Could you check a few things on this model? Use its own coordinates, in mm. A direction names the side the tool comes from. Give positions to 0.01 mm unless a question says otherwise; leave off trailing zeros. Loops run counter-clockwise (first coordinate to the right, second up) from the corner with the lowest first, then second, coordinate; pieces in that order, holes last. Notation, with made-up numbers: M 48.25,43 L 67.25,43 A21 ccw 67.25,69 Z; hole C 18.25,8 d11. An arc over 180 degrees is marked long. Use a Markdown table: item, result. Add a question column.
1) Suppose I cut it at D-D on z = -27. List the corners of the cut face in (x, y) for me.
2) Suppose I cut it at B-B on y = 17.5. List the corners of the cut face in (x, z) for me, and give its area (3 significant figures).
3) Suppose I cut it at A-A on x = -52.5. List the corners of the cut face in (y, z) for me.
4) We'd pull the mould along Z, two halves only. Please class faces 1 (the flat face through (63, 88, 0)), 2 (the flat face through (-105, 11, 8)), 3 (the cylindrical face through (-80, 55, 0)), 4 (the flat face through (-39, 2, 0)): +Z half, -Z half, draft (parallel to the pull), parting line (faces both ways), or undercut.
5) If I drill on line 1 along X through (y, z) = (7, 0); line 2 along Z through (x, y) = (52, 11); line 3 along Y through (x, z) = (-103.5, 21.5), over which ranges is the centre line in solid material (lowest first)? Write a range as [from, to].
6) Will these pins go through, and if not, where does the flat tip stop? pin 1 Ø6 at (y, z) = (54.5, 13.5) entering from +X; pin 2 Ø3 at (x, z) = (-33.5, -5) entering from +Y; pin 3 Ø1.5 at (x, z) = (-81, -0.5) entering from +Y; pin 4 Ø5.5 at (x, z) = (0, 0) entering from -Y.
7) Suppose I cut it at C-C on y = 38. List the corners of the cut face in (x, z) for me.
8) Which directions (+Z, -Z, +X, -X, +Y, -Y) give clear straight access to the entire face, cutting with the end or side of a thin tool? Please do faces 5 (the flat face through (-2, 24, 32)), 6 (the flat face through (5, 31, -20)), 7 (the cylindrical face through (80, 55, 0)), 8 (the cylindrical face through (94, 11, 0)), 9 (the flat face through (-36, 76, 0)).
```python
from build123d import *

# Parameters (mm, degrees)
SKETCH1_W               = 260
SKETCH1_H               = 64
BOSS_EXTRUDE1_DEPTH     = 22
SKETCH3_R               = 9.5
BOSS_EXTRUDE2_DEPTH     = 66
CUT_EXTRUDE2_DEPTH      = 75
CUT_EXTRUDE3_DEPTH      = 20
CUT_EXTRUDE5_DEPTH      = 40
CUT_EXTRUDE5_DEPTH_BACK = 6
SKETCH7_R               = 3
SKETCH8_W               = 67.321211119
SKETCH8_H               = 40
CUT_EXTRUDE6_DEPTH      = 2
SKETCH9_R               = 9.5
CUT_EXTRUDE7_DEPTH      = 45


with BuildPart() as part:
    # Sketch1 → Boss-Extrude1 (new body)
    with BuildSketch(Plane(origin=(0, 0, 0), x_dir=(1, 0, 0), z_dir=(0, 1, 0))):
        Rectangle(SKETCH1_W, SKETCH1_H)
        with BuildLine():
            Line((-102, -8), (-108, -8))
            ThreePointArc((-108, -8), (-116, 0), (-108, 8))
            Line((-108, 8), (-102, 8))
            ThreePointArc((-102, 8), (-94, 0), (-102, -8))
        make_face(mode=Mode.SUBTRACT)
        with BuildLine():
            Line((102, -8), (108, -8))
            ThreePointArc((108, -8), (116, 0), (108, 8))
            Line((108, 8), (102, 8))
            ThreePointArc((102, 8), (94, 0), (102, -8))
        make_face(mode=Mode.SUBTRACT)
    extrude(amount=BOSS_EXTRUDE1_DEPTH)

    # Sketch3 → Boss-Extrude2 (add)
    with BuildSketch(Plane(origin=(0, 88, 0), x_dir=(-1, 0, 0), z_dir=(0, -1, 0))):
        with BuildLine():
            Line((73.321211119, -32), (-73.321211119, -32))
            ThreePointArc((-73.321211119, -32), (-80, 0), (-73.321211119, 32))
            Line((-73.321211119, 32), (73.321211119, 32))
            ThreePointArc((73.321211119, 32), (80, 0), (73.321211119, -32))
        make_face()
        with Locations(Location((-52.5, 0, 0), (0, 0, 270))):
            Circle(SKETCH3_R, mode=Mode.SUBTRACT)
        with Locations(Location((52.5, 0, 0), (0, 0, 270))):
            Circle(SKETCH3_R, mode=Mode.SUBTRACT)
    extrude(amount=BOSS_EXTRUDE2_DEPTH)

    # Sketch5 → Cut-Extrude2 (cut)
    with BuildSketch(Plane.XY.offset(32)):
        with BuildLine():
            Line((-36, 63), (-32, 63))
            ThreePointArc((-32, 63), (-22.627416998, 40.372583002), (0, 31))
            Line((0, 31), (0, 88))
            Line((0, 88), (-36, 88))
            Line((-36, 88), (-36, 63))
        make_face()
    cut_extrude2 = extrude(amount=-CUT_EXTRUDE2_DEPTH, mode=Mode.SUBTRACT)

    # Sketch6 → Cut-Extrude3 (cut, symmetric)
    with BuildSketch(Plane.XY):
        with BuildLine():
            Line((-34, 63), (0, 63))
            Line((0, 63), (0, 29))
            ThreePointArc((0, 29), (-24.04163056, 38.95836944), (-34, 63))
        make_face()
    cut_extrude3 = extrude(amount=CUT_EXTRUDE3_DEPTH, both=True, mode=Mode.SUBTRACT)

    # Mirror1: Cut-Extrude2, Cut-Extrude3 across plane
    add(cut_extrude2.mirror(Plane(origin=(0, 0, 0), x_dir=(0, 0, 1), z_dir=(1, 0, 0))), mode=Mode.SUBTRACT)
    add(cut_extrude3.mirror(Plane(origin=(0, 0, 0), x_dir=(0, 0, 1), z_dir=(1, 0, 0))), mode=Mode.SUBTRACT)

    # Sketch7 → Cut-Extrude5 (cut, two sides: drawn at the far end of the back side and taken through both)
    with BuildSketch(Plane(origin=(0, 29, 0), x_dir=(1, 0, 0), z_dir=(0, 1, 0)).offset(-CUT_EXTRUDE5_DEPTH_BACK)):
        with Locations(Location((0, 0, 0), (0, 0, 90))):
            Circle(SKETCH7_R)
    extrude(amount=CUT_EXTRUDE5_DEPTH + CUT_EXTRUDE5_DEPTH_BACK, mode=Mode.SUBTRACT)

    # Sketch8 → Cut-Extrude6 (cut)
    with BuildSketch(Plane.XZ):
        with Locations((39.66060556, 0)):
            Rectangle(SKETCH8_W, SKETCH8_H)
    cut_extrude6 = extrude(amount=-CUT_EXTRUDE6_DEPTH, mode=Mode.SUBTRACT)

    # Mirror2: Cut-Extrude6 across plane
    add(cut_extrude6.mirror(Plane(origin=(0, 0, 0), x_dir=(0, 0, 1), z_dir=(1, 0, 0))), mode=Mode.SUBTRACT)

    # Sketch9 → Cut-Extrude7 (cut)
    with BuildSketch(Plane(origin=(0, 22, 0), x_dir=(1, 0, 0), z_dir=(0, 1, 0))):
        with Locations(Location((-52.5, 0, 0), (0, 0, 270))):
            Circle(SKETCH9_R)
        with Locations(Location((52.5, 0, 0), (0, 0, 270))):
            Circle(SKETCH9_R)
    extrude(amount=-CUT_EXTRUDE7_DEPTH, mode=Mode.SUBTRACT)


solid = part.part
```
Answer block:
| question | item | result |
|---|---|---|
| 1 | outline | M -130,0 L 130,0 L 130,22 L 75.31,22 L 75.31,88 L 36,88 L 36,63 L 32,63 A32 cw -32,63 L -36,63 L -36,88 L -75.31,88 L -75.31,22 L -130,22 Z |
| 2 | outline | M -130,-32 L 130,-32 L 130,32 L -130,32 Z; hole M -108,-8 L -102,-8 A8 ccw -102,8 L -108,8 A8 ccw Z; hole C -52.5,0 d19; hole C 52.5,0 d19; hole M 102,-8 L 108,-8 A8 ccw 108,8 L 102,8 A8 ccw Z |
| 2 | area | 15,500 mm^2 |
| 3 | outline | M 0,-32 L 88,-32 L 88,-9.5 L 2,-9.5 L 2,-20 L 0,-20 Z; M 0,20 L 2,20 L 2,9.5 L 88,9.5 L 88,32 L 0,32 Z |
| 4 | face 1 | draft |
| 4 | face 2 | undercut |
| 4 | face 3 | parting line |
| 4 | face 4 | undercut |
| 5 | line 1 | x = [-130, -116], [-94, -62], [-43, 43], [62, 94], [116, 130] |
| 5 | line 2 | z = [-32, -9.49], [9.49, 32] |
| 5 | line 3 | y = [0, 22] |
| 6 | pin 1 | stops at x = 79.31 |
| 6 | pin 2 | stops at y = 63 |
| 6 | pin 3 | stops at y = 22 |
| 6 | pin 4 | stops at y = 0 |
| 7 | outline | M -73.32,-32 L -19.97,-32 L -19.97,-20 L -23.04,-20 L -23.04,20 L -19.97,20 L -19.97,32 L -73.32,32 A80 ccw Z; M 19.97,-32 L 73.32,-32 A80 ccw 73.32,32 L 19.97,32 L 19.97,20 L 23.04,20 L 23.04,-20 L 19.97,-20 Z; hole C -52.5,0 d19; hole C 52.5,0 d19 |
| 8 | face 5 | +Z, +X, -X, +Y, -Y |
| 8 | face 6 | +Y |
| 8 | face 7 | +X, +Y |
| 8 | face 8 | +Y, -Y |
| 8 | face 9 | +Z, -Z, +Y |
